```python
from build123d import *

# Parameters (mm, degrees)
SKETCH1_W           = 11.5
SKETCH1_H           = 6.18
SKETCH1_W_2         = 8.5
SKETCH1_H_2         = 3.18
BOSS_EXTRUDE1_DEPTH = 4.88
SKETCH2_W           = 11.5
SKETCH2_H           = 6.18
BOSS_EXTRUDE2_DEPTH = 1
SKETCH3_W           = 4.16
SKETCH3_H           = 6.18
BOSS_EXTRUDE3_DEPTH = 4.25
SKETCH4_R           = 1.47
CUT_EXTRUDE1_DEPTH  = 7.5
SKETCH5_R           = 1.47
CUT_EXTRUDE2_DEPTH  = 14.480166913


with BuildPart() as part:
    # Sketch1 → Boss-Extrude1 (new body)
    with BuildSketch(Plane.XY):
        with Locations((4.25, 1.59)):
            Rectangle(SKETCH1_W, SKETCH1_H)
        with Locations((4.25, 1.59)):
            Rectangle(SKETCH1_W_2, SKETCH1_H_2, mode=Mode.SUBTRACT)
    extrude(amount=BOSS_EXTRUDE1_DEPTH)

    # Sketch2 → Boss-Extrude2 (add)
    with BuildSketch(Plane(origin=(0, 0, 0), x_dir=(-1, 0, 0), z_dir=(0, 0, -1))):
        with Locations((-4.25, 1.59)):
            Rectangle(SKETCH2_W, SKETCH2_H)
    extrude(amount=BOSS_EXTRUDE2_DEPTH)

    # Sketch3 → Boss-Extrude3 (add)
    with BuildSketch(Plane(origin=(0, 0, -1), x_dir=(-1, 0, 0), z_dir=(0, 0, -1))):
        with Locations((-7.92, 1.59)):
            Rectangle(SKETCH3_W, SKETCH3_H)
        with Locations((-0.58, 1.59)):
            Rectangle(SKETCH3_W, SKETCH3_H)
    extrude(amount=BOSS_EXTRUDE3_DEPTH)

    # Sketch4 → Cut-Extrude1 (cut)
    with BuildSketch(Plane(origin=(10, 0, 0), x_dir=(0, 0, -1), z_dir=(1, 0, 0))):
        with Locations((3, 1.59)):
            Circle(SKETCH4_R)
    extrude(amount=-CUT_EXTRUDE1_DEPTH, mode=Mode.SUBTRACT)

    # Sketch5 → Cut-Extrude2 (cut, through all)
    with BuildSketch(Plane.ZY.offset(1.5)):
        with Locations(Location((-3, 1.59, 0), (0, 0, 270))):
            Circle(SKETCH5_R)
    extrude(amount=-CUT_EXTRUDE2_DEPTH, mode=Mode.SUBTRACT)


solid = part.part
```
For this review, take the finished solid that the model builds, in its own axes (mm). A direction names the side the tool comes from. Round coordinates to 2 decimals unless told otherwise and drop trailing zeros. Write each loop counter-clockwise with the first axis right and the second up, starting at its lowest first coordinate (ties: lowest second). Pieces come first, ordered by that corner, then holes. Notation, with made-up numbers: (10, 37.5) - (41, 37.5) arc R15 ccw to (41, 56.5) - close; hole circle Ø3 at (-14, 36). An arc over 180 degrees is marked (long way). Use CSV: the item, a comma, the result in double quotes.
1) For faces 1 (the flat face through (8.5, 2, 2)), 2 (the flat face through (4, 2, -1)), 3 (the flat face through (1, 2, -5.25)), list the 3-axis set-ups (+Z, -Z, +X, -X, +Y, -Y) from which the entire face can be reached by the end or side of a thin tool; tool diameter is ignored.
Conclusion:
face 1,"+Z"
face 2,"-Z, +Y, -Y"
face 3,"-Z, +X, -X, +Y, -Y"
2) The part is to be moulded in two halves that separate along X. For faces 4 (the flat face through (-1.5, 2, 0)), 5 (the flat face through (4, 2, 0)), 6 (the flat face through (4, -1.5, 0)), say which applies: pulls with the +X half, pulls with the -X half, needs draft (parallel to the pull), parting line crosses it, or undercut.
Conclusion:
face 4,"pulls with the -X half"
face 5,"undercut"
face 6,"needs draft"
3) Wall thickness on line 1 along Y through (x, z) = (8.9, -3); line 2 along Y through (x, z) = (0.75, 3.5); line 3 along Z through (x, y) = (7.45, 1.59): over which ranges is each line inside the solid? List them lowest first. Write a range as from..to.
Conclusion:
line 1,"y = -1.5..0.12, 3.06..4.68"
line 2,"y = -1.5..0, 3.18..4.68"
line 3,"z = -5.25..-4.47, -1.53..0"
4) Add section B-B on z = -2.25. Write out the cut boundary in (x, y).
Conclusion:
outline,"(-1.5, -1.5) - (2.66, -1.5) - (2.66, 0.33) - (-1.5, 0.33) - close; (-1.5, 2.85) - (2.66, 2.85) - (2.66, 4.68) - (-1.5, 4.68) - close; (5.84, -1.5) - (10, -1.5) - (10, 0.33) - (5.84, 0.33) - close; (5.84, 2.85) - (10, 2.85) - (10, 4.68) - (5.84, 4.68) - close"
5) Add section D-D on z = 4.25. Write out the cut boundary in (x, y).
Conclusion:
outline,"(-1.5, -1.5) - (10, -1.5) - (10, 4.68) - (-1.5, 4.68) - close; hole (0, 0) - (8.5, 0) - (8.5, 3.18) - (0, 3.18) - close"
6) Add section A-A on y = 1. Write out the cut boundary in (x, z), and give its area (3 significant figures).
Conclusion:
outline,"(-1.5, -5.25) - (2.66, -5.25) - (2.66, -4.35) - (-1.5, -4.35) - close; (-1.5, -1.65) - (2.66, -1.65) - (2.66, -1) - (5.84, -1) - (5.84, -1.65) - (10, -1.65) - (10, 4.88) - (8.5, 4.88) - (8.5, 0) - (0, 0) - (0, 4.88) - (-1.5, 4.88) - close; (5.84, -5.25) - (10, -5.25) - (10, -4.35) - (5.84, -4.35) - close"
area,"39.1 mm^2"
7) Add section C-C on x = 1.5. Write out the cut boundary in (y, z), and give its area (3 significant figures).
Conclusion:
outline,"(-1.5, -5.25) - (4.68, -5.25) - (4.68, 4.88) - (3.18, 4.88) - (3.18, 0) - (0, 0) - (0, 4.88) - (-1.5, 4.88) - close; hole circle Ø2.94 at (1.59, -3)"
area,"40.3 mm^2"
8) Clearance check with a flat-ended pin moving along its axis: pin 1 Ø1.6 at (x, y) = (4, 0.5) entering from -Z. State where the tip first meets the part, or that it passes through.
Conclusion:
pin 1,"stops at z = -1"
